Can you work these out from the model? Positions are in its coordinate system, mm. A direction names the side the tool comes from. Coordinates: 2 decimals unless noted, no trailing zeros. Order: outer loops, then holes, each group sorted by start corner. A loop starts at its lowest first (then second) coordinate and runs counter-clockwise, first axis right, second up. Notation, with made-up numbers: (0, 53.5) - (29, 53.5) arc R22 cw to (29, 67.5) - close; hole circle Ø4 at (53.25, 42.25). An arc over 180 degrees is marked (long way). Return JSON: item names as keys, results as strings. Group by question number.
1) If I drill on line 1 along X through (y, z) = (6.75, 9.5); line 2 along X through (y, z) = (1.75, -7.5); line 3 along Z through (x, y) = (16.5, -2.25), over which ranges is the centre line in solid material (lowest first)?
2) If we mould it in two halves opening along Z, with no side actions, what happens to faces 1 (the face through (1.733, 3.591, -19.135)), 2 (the face through (-10, -8, 5))? For each: pulls with the +Z half, pulls with the -Z half, needs draft (parallel to the pull), parting line crosses it, or undercut.
3) Imagine slicing it at A-A (y = -6). Write out the boundary of the cut face in (x, z), and give its area (3 significant figures).
4) For pin 1 Ø4.5 at (x, z) = (-15.18, -7.07) entering from -Y; pin 2 Ø5 at (x, y) = (-18, 4.5) entering from +Z; pin 3 Ø5 at (x, y) = (-14, 5) entering from -Z; pin 4 Ø4.5 at (x, z) = (-0.5, -16) entering from +Y, each with a flat end and sliding along its axis, tell me the tip position at first contact or that it passes through.
5) Which directions (+Z, -Z, +X, -X, +Y, -Y) give clear straight access to the entire face, cutting with the end or side of a thin tool? Please do faces 3 (the face through (2.38, 0.87, 10.74)), 4 (the face through (-0.9, 3.6, -12.7)).
6) Imagine slicing it at B-B (y = 8.75). Give the number of separate pieces and of enclosed holes in the cut face, and give its area (3 significant figures).
```python
from build123d import *

# Parameters (mm, degrees)
SKETCH1_R               = 11
BOSS_EXTRUDE1_DEPTH     = 10
SKETCH2_R               = 32.5
SKETCH3_R               = 23.5
SKETCH3_4_R             = 11
CUT_EXTRUDE1_DEPTH      = 1.0000001
CUT_EXTRUDE1_DEPTH_BACK = 19
CUT_EXTRUDE2_DEPTH      = 13
SKETCH1_7_R             = 2.75
CUT_EXTRUDE3_DEPTH      = 9.0000001


with BuildPart() as part:
    # Sketch1 → Boss-Extrude1 (new body)
    with BuildSketch(Plane(origin=(0, 0, 0), x_dir=(1, 0, 0), z_dir=(0, 1, 0))):
        with BuildLine():
            ThreePointArc((27.993478679, -0.604277614), (26.22801827, 1.074037998), (27.850343554, 2.891083518))
            ThreePointArc((27.850343554, 2.891083518), (27.77024444, 3.579598264), (27.673126544, 4.26591928))
            ThreePointArc((27.673126544, 4.26591928), (25.643050997, 5.612168524), (26.925202872, 7.683322869))
            ThreePointArc((26.925202872, 7.683322869), (26.726761313, 8.347468463), (26.511940461, 9.006498375))
            ThreePointArc((26.511940461, 9.006498375), (24.278932596, 9.979776149), (25.181953525, 12.242108342))
            ThreePointArc((25.181953525, 12.242108342), (24.871199067, 12.861705057), (24.545202484, 13.473419575))
            ThreePointArc((24.545202484, 13.473419575), (22.177111114, 14.044153326), (22.673563263, 16.428923548))
            ThreePointArc((22.673563263, 16.428923548), (22.259938023, 16.985145252), (21.832670949, 17.530957739))
            ThreePointArc((21.832670949, 17.530957739), (19.401449332, 17.681806011), (19.476248255, 20.116554226))
            ThreePointArc((19.476248255, 20.116554226), (18.972320026, 20.592500403), (18.456764755, 21.055826623))
            ThreePointArc((18.456764755, 21.055826623), (16.036284331, 20.782205967), (15.687157298, 23.192953583))
            ThreePointArc((15.687157298, 23.192953583), (15.108237686, 23.574162849), (14.520059104, 23.940924869))
            ThreePointArc((14.520059104, 23.940924869), (12.183864944, 23.251149112), (11.421420006, 25.564646781))
            ThreePointArc((11.421420006, 25.564646781), (10.785099188, 25.839536286), (10.142168805, 26.098590229))
            ThreePointArc((10.142168805, 26.098590229), (7.961244987, 25.013617856), (6.808648646, 27.159571124))
            ThreePointArc((6.808648646, 27.159571124), (6.13426091, 27.319788489), (5.456113839, 27.463263131))
            ThreePointArc((5.456113839, 27.463263131), (3.496726629, 26.01606048), (1.988999942, 27.929265641))
            ThreePointArc((1.988999942, 27.929265641), (1.297036218, 27.969942743), (0.604277614, 27.993478679))
            ThreePointArc((0.604277614, 27.993478679), (-1.074037998, 26.22801827), (-2.891083518, 27.850343554))
            ThreePointArc((-2.891083518, 27.850343554), (-3.579598264, 27.77024444), (-4.26591928, 27.673126544))
            ThreePointArc((-4.26591928, 27.673126544), (-5.612168524, 25.643050997), (-7.683322869, 26.925202872))
            ThreePointArc((-7.683322869, 26.925202872), (-8.347468463, 26.726761313), (-9.006498375, 26.511940461))
            ThreePointArc((-9.006498375, 26.511940461), (-9.979776149, 24.278932596), (-12.242108342, 25.181953525))
            ThreePointArc((-12.242108342, 25.181953525), (-12.861705057, 24.871199067), (-13.473419575, 24.545202484))
            ThreePointArc((-13.473419575, 24.545202484), (-14.044153326, 22.177111114), (-16.428923548, 22.673563263))
            ThreePointArc((-16.428923548, 22.673563263), (-16.985145252, 22.259938023), (-17.530957739, 21.832670949))
            ThreePointArc((-17.530957739, 21.832670949), (-17.681806011, 19.401449332), (-20.116554226, 19.476248255))
            ThreePointArc((-20.116554226, 19.476248255), (-20.592500403, 18.972320026), (-21.055826623, 18.456764755))
            ThreePointArc((-21.055826623, 18.456764755), (-20.782205967, 16.036284331), (-23.192953583, 15.687157299))
            ThreePointArc((-23.192953583, 15.687157299), (-23.574162849, 15.108237686), (-23.940924869, 14.520059104))
            ThreePointArc((-23.940924869, 14.520059104), (-23.251149112, 12.183864944), (-25.564646781, 11.421420006))
            ThreePointArc((-25.564646781, 11.421420006), (-25.839536286, 10.785099188), (-26.098590229, 10.142168805))
            ThreePointArc((-26.098590229, 10.142168805), (-25.013617856, 7.961244987), (-27.159571124, 6.808648646))
            ThreePointArc((-27.159571124, 6.808648646), (-27.319788489, 6.13426091), (-27.463263131, 5.456113839))
            ThreePointArc((-27.463263131, 5.456113839), (-26.01606048, 3.496726629), (-27.929265641, 1.988999942))
            ThreePointArc((-27.929265641, 1.988999942), (-27.969942743, 1.297036218), (-27.993478679, 0.604277614))
            ThreePointArc((-27.993478679, 0.604277614), (-26.22801827, -1.074037998), (-27.850343554, -2.891083518))
            ThreePointArc((-27.850343554, -2.891083518), (-27.77024444, -3.579598264), (-27.673126544, -4.26591928))
            ThreePointArc((-27.673126544, -4.26591928), (-25.643050997, -5.612168524), (-26.925202872, -7.683322869))
            ThreePointArc((-26.925202872, -7.683322869), (-26.726761313, -8.347468463), (-26.511940461, -9.006498375))
            ThreePointArc((-26.511940461, -9.006498375), (-24.278932596, -9.979776149), (-25.181953525, -12.242108342))
            ThreePointArc((-25.181953525, -12.242108342), (-24.871199067, -12.861705057), (-24.545202484, -13.473419575))
            ThreePointArc((-24.545202484, -13.473419575), (-22.177111114, -14.044153326), (-22.673563263, -16.428923548))
            ThreePointArc((-22.673563263, -16.428923548), (-22.259938023, -16.985145252), (-21.832670949, -17.530957739))
            ThreePointArc((-21.832670949, -17.530957739), (-19.401449332, -17.681806011), (-19.476248255, -20.116554226))
            ThreePointArc((-19.476248255, -20.116554226), (-18.972320026, -20.592500403), (-18.456764755, -21.055826623))
            ThreePointArc((-18.456764755, -21.055826623), (-16.036284331, -20.782205967), (-15.687157298, -23.192953583))
            ThreePointArc((-15.687157298, -23.192953583), (-15.108237686, -23.574162849), (-14.520059104, -23.940924869))
            ThreePointArc((-14.520059104, -23.940924869), (-12.183864944, -23.251149112), (-11.421420006, -25.564646781))
            ThreePointArc((-11.421420006, -25.564646781), (-10.785099188, -25.839536286), (-10.142168805, -26.098590229))
            ThreePointArc((-10.142168805, -26.098590229), (-7.961244987, -25.013617856), (-6.808648646, -27.159571124))
            ThreePointArc((-6.808648646, -27.159571124), (-6.13426091, -27.319788489), (-5.456113839, -27.463263131))
            ThreePointArc((-5.456113839, -27.463263131), (-3.496726629, -26.01606048), (-1.988999942, -27.929265641))
            ThreePointArc((-1.988999942, -27.929265641), (-1.297036218, -27.969942743), (-0.604277614, -27.993478679))
            ThreePointArc((-0.604277614, -27.993478679), (1.074037998, -26.22801827), (2.891083518, -27.850343554))
            ThreePointArc((2.891083518, -27.850343554), (3.579598264, -27.77024444), (4.26591928, -27.673126544))
            ThreePointArc((4.26591928, -27.673126544), (5.612168524, -25.643050997), (7.683322869, -26.925202872))
            ThreePointArc((7.683322869, -26.925202872), (8.347468463, -26.726761312), (9.006498375, -26.511940461))
            ThreePointArc((9.006498375, -26.511940461), (9.979776149, -24.278932596), (12.242108342, -25.181953525))
            ThreePointArc((12.242108342, -25.181953525), (12.861705057, -24.871199067), (13.473419575, -24.545202484))
            ThreePointArc((13.473419575, -24.545202484), (14.044153326, -22.177111114), (16.428923548, -22.673563263))
            ThreePointArc((16.428923548, -22.673563263), (16.985145252, -22.259938023), (17.530957739, -21.832670949))
            ThreePointArc((17.530957739, -21.832670949), (17.681806011, -19.401449332), (20.116554226, -19.476248255))
            ThreePointArc((20.116554226, -19.476248255), (20.592500403, -18.972320026), (21.055826623, -18.456764755))
            ThreePointArc((21.055826623, -18.456764755), (20.782205967, -16.036284331), (23.192953583, -15.687157298))
            ThreePointArc((23.192953583, -15.687157298), (23.574162849, -15.108237686), (23.940924869, -14.520059104))
            ThreePointArc((23.940924869, -14.520059104), (23.251149112, -12.183864944), (25.564646781, -11.421420006))
            ThreePointArc((25.564646781, -11.421420006), (25.839536286, -10.785099188), (26.098590229, -10.142168805))
            ThreePointArc((26.098590229, -10.142168805), (25.013617856, -7.961244987), (27.159571124, -6.808648646))
            ThreePointArc((27.159571124, -6.808648646), (27.319788489, -6.13426091), (27.463263131, -5.456113839))
            ThreePointArc((27.463263131, -5.456113839), (26.01606048, -3.496726629), (27.929265641, -1.988999942))
            ThreePointArc((27.929265641, -1.988999942), (27.969942743, -1.297036218), (27.993478679, -0.604277614))
        make_face()
        Circle(SKETCH1_R, mode=Mode.SUBTRACT)
    extrude(amount=BOSS_EXTRUDE1_DEPTH)

    # Sketch2 → Loft2 section 0
    with BuildSketch(Plane.XZ):
        Circle(SKETCH2_R)
    # Sketch3 → Loft2 section 1
    with BuildSketch(Plane(origin=(0, -8, 0), x_dir=(-1, 0, 0), z_dir=(0, -1, 0))):
        Circle(SKETCH3_R)
    loft()

    # Sketch3<4> → Cut-Extrude1 (cut, two sides)
    with BuildSketch(Plane(origin=(0, -8, 0), x_dir=(-1, 0, 0), z_dir=(0, -1, 0))) as cut_extrude1_sk:
        Circle(SKETCH3_4_R)
    extrude(amount=CUT_EXTRUDE1_DEPTH, mode=Mode.SUBTRACT)
    extrude(cut_extrude1_sk.sketch, amount=-CUT_EXTRUDE1_DEPTH_BACK, mode=Mode.SUBTRACT)

    # Sketch4 → Cut-Extrude2 (cut)
    with BuildSketch(Plane(origin=(0, 10, 0), x_dir=(1, 0, 0), z_dir=(0, 1, 0))):
        Polygon((-10.576848295, 7.715277219), (-13.434334579, 11.383692699), (-18.040018719, 10.743244726), (-19.788216575, 6.434381273), (-16.93073029, 2.765965793), (-12.325046151, 3.406413766), align=None)
        Polygon((-18.323932212, -10.251492132), (-15.466445928, -13.919907613), (-10.860761788, -13.27945964), (-9.112563932, -8.970596187), (-11.970050217, -5.302180706), (-16.575734356, -5.942628679), align=None)
        Polygon((1.393201921, 13.017457925), (3.141399777, 17.326321378), (0.283913493, 20.994736859), (-4.321770647, 20.354288886), (-6.069968503, 16.045425433), (-3.212482218, 12.377009952), align=None)
        Polygon((11.970050217, 5.302180706), (16.575734356, 5.942628679), (18.323932212, 10.251492132), (15.466445928, 13.919907613), (10.860761788, 13.27945964), (9.112563932, 8.970596187), align=None)
        Polygon((10.576848295, -7.715277219), (13.434334579, -11.383692699), (18.040018719, -10.743244726), (19.788216575, -6.434381273), (16.93073029, -2.765965793), (12.325046151, -3.406413766), align=None)
        Polygon((-1.393201921, -13.017457925), (-3.141399777, -17.326321378), (-0.283913493, -20.994736859), (4.321770647, -20.354288886), (6.069968503, -16.045425433), (3.212482218, -12.377009952), align=None)
    extrude(amount=-CUT_EXTRUDE2_DEPTH, mode=Mode.SUBTRACT)

    # Sketch1<7> → Cut-Extrude3 (cut, through all)
    with BuildSketch(Plane(origin=(0, 0, 0), x_dir=(1, 0, 0), z_dir=(0, 1, 0))):
        with Locations((15.182532435, -7.074829246)):
            Circle(SKETCH1_7_R)
        with Locations((1.464284363, -16.685873406)):
            Circle(SKETCH1_7_R)
        with Locations((-13.718248072, -9.611044159)):
            Circle(SKETCH1_7_R)
        with Locations((-15.182532435, 7.074829246)):
            Circle(SKETCH1_7_R)
        with Locations((-1.464284363, 16.685873406)):
            Circle(SKETCH1_7_R)
        with Locations((13.718248072, 9.611044159)):
            Circle(SKETCH1_7_R)
    extrude(amount=-CUT_EXTRUDE3_DEPTH, mode=Mode.SUBTRACT)


solid = part.part
```
Calculated:
{
 "1": {"line 1": "-24.57 to -18.02, -9.33 to -5.55, 5.55 to 11.97, 18.54 to 25.25", "line 2": "-25.24 to -19.36, -10.66 to -8.05, 8.05 to 10.26, 17.21 to 26.47", "line 3": "-25.02 to -12.59, -5.93 to 2.83, 10.96 to 25.02"},
 "2": {"face 1": "undercut", "face 2": "needs draft"},
 "3": {"outline": "circle Ø51.5 at (0, 0); hole circle Ø5.5 at (-15.18, -7.07); hole circle Ø5.5 at (-13.72, 9.61); hole circle Ø22 at (0, 0); hole circle Ø5.5 at (-1.46, -16.69); hole circle Ø5.5 at (1.46, 16.69); hole circle Ø5.5 at (13.72, -9.61); hole circle Ø5.5 at (15.18, 7.07)", "area": "1,560 mm2"},
 "4": {"pin 1": "through", "pin 2": "z = 23.32", "pin 3": "z = -25.18", "pin 4": "y = -3"},
 "5": {"face 3": "+Y, -Y", "face 4": "+Y"},
 "6": {"separate pieces": "1", "enclosed holes": "7", "area": "1,570 mm2"}
}
